Print and shaded views of the part. All mm, measured from the part's lowest x, y and z. A direction names the side the tool comes from. Coordinates: 2 decimals unless noted, no trailing zeros. Order: outer loops, then holes, each group sorted by start corner. A loop starts at its lowest first (then second) coordinate and runs counter-clockwise, first axis right, second up. Notation, with made-up numbers: (51, 21) - (100, 21) arc R23 ccw to (100, 54) - close; hole circle Ø6 at (4, -39). An arc over 180 degrees is marked (long way). Write each question's results on one line, items separated by ' | '.
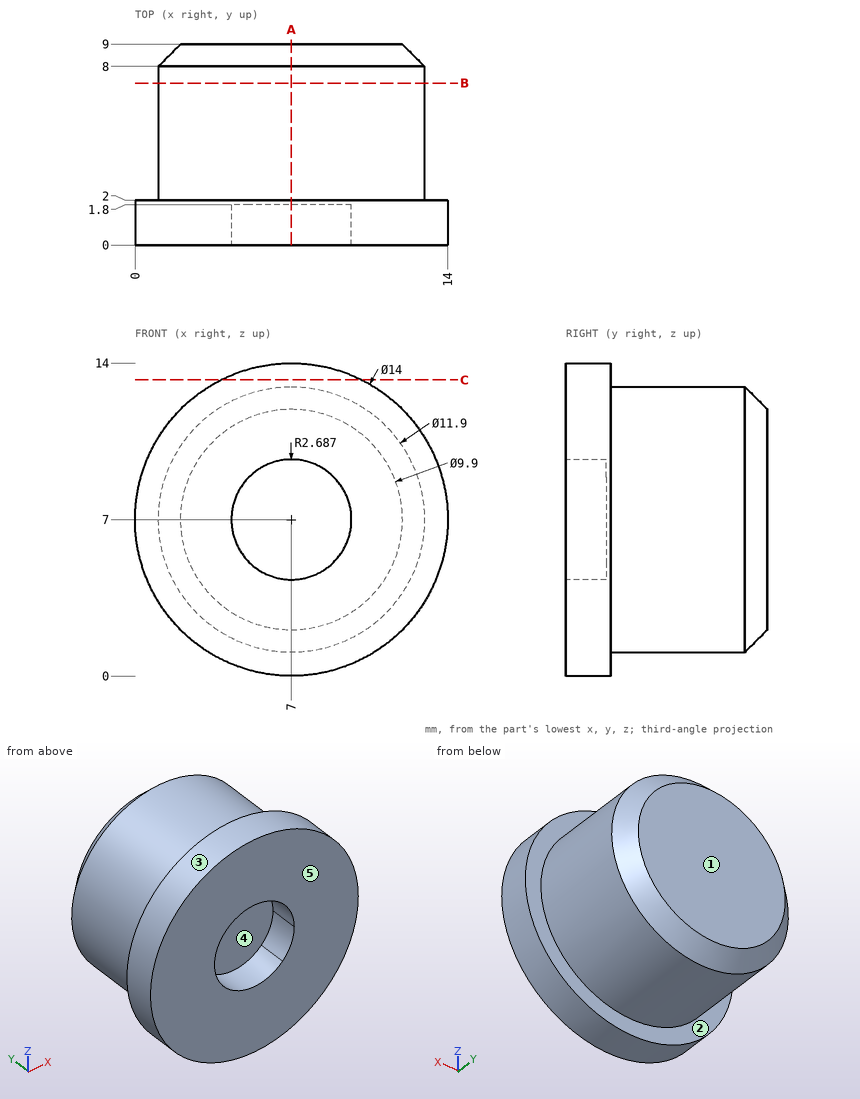
1. Band-saw the part on A-A on x = 7. Give the cut face in (y, z), then the cut area to 3 significant figures.
Solved:
outline: (0, 0) - (2, 0) - (2, 1.05) - (8, 1.05) - (9, 2.05) - (9, 11.95) - (8, 12.95) - (2, 12.95) - (2, 14) - (0, 14) - (0, 9.69) - (1.8, 9.69) - (1.8, 4.31) - (0, 4.31) - close | area: 101 mm2
2. Probe line 1 (Y direction, x = 10, z = 1.25); line 2 (X direction, y = 1.25, z = 5.5); line 3 (Y direction, x = 9, z = 6.25). List the from-to ranges inside material, lowest first.
Solved:
line 1: y = 0 to 2 | line 2: x = 0.16 to 4.77, 9.23 to 13.84 | line 3: y = 1.8 to 9
3. Band-saw the part on B-B on y = 7.25. Give the cut face in (x, z).
Solved:
outline: circle Ø11.9 at (7, 7)
4. Tool access for the marked faces 1 and 2: list every direction of +Z, -Z, +X, -X, +Y, -Y with a clear straight run to the whole face (end or side of a thin tool).
Solved:
face 1: +Z, -Z, +X, -X, +Y | face 2: +Y
5. Band-saw the part on C-C on z = 13.25. Give the cut face in (x, y), then the cut area to 3 significant figures.
Solved:
outline: (3.85, 0) - (10.15, 0) - (10.15, 2) - (3.85, 2) - close | area: 12.6 mm2
6. Drop flat-ended pins along their axis: pin 1 Ø3 at (x, z) = (7.5, 7.5) entering from -Y; pin 2 Ø1.5 at (x, y) = (4, 2.5) entering from -Z; pin 3 Ø1.5 at (y, z) = (1, 4) entering from -X. Give the stop position or say it passes through.
Solved:
pin 1: stops at y = 1.8 | pin 2: stops at z = 0.44 | pin 3: stops at x = 0.37
7. Two-plate mould, pull along Z, no slides. Class the marked faces 3, 4 and 5: +Z half, -Z half, draft (parallel to the pull), parting line (faces both ways), or undercut.
Solved:
face 3: parting line | face 4: undercut | face 5: draft
